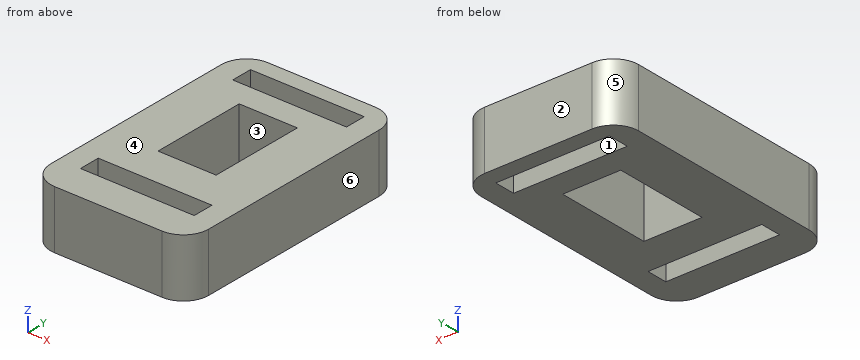
```python
from build123d import *

# Parameters (mm, degrees)
F1_DEPTH = 5.842
F2_W     = 5.842
F2_H     = 9.6774
F2_W_2   = 11.43
F2_H_2   = 2.116666
F2_H_3   = 2.116667
F3_DEPTH = 5.842


with BuildPart() as f1:
    # F0 (on Top) → F1 (new body)
    with BuildSketch(Plane.XY):
        with BuildLine():
            Line((4.632767, -11.371723), (-6.162233, -11.371723))
            ThreePointArc((-6.162233, -11.371723), (-7.958284, -12.115671), (-8.702233, -13.911723))
            Line((-8.702233, -13.911723), (-8.702233, -34.231723))
            ThreePointArc((-8.702233, -34.231723), (-7.958284, -36.027774), (-6.162233, -36.771723))
            Line((-6.162233, -36.771723), (4.632767, -36.771723))
            ThreePointArc((4.632767, -36.771723), (6.428818, -36.027774), (7.172767, -34.231723))
            Line((7.172767, -34.231723), (7.172767, -13.911723))
            ThreePointArc((7.172767, -13.911723), (6.428818, -12.115671), (4.632767, -11.371723))
        make_face()
    extrude(amount=-F1_DEPTH)

    # F2 (on Top) → F3 (cut, through all)
    with BuildSketch(Plane.XY):
        with Locations((-0.764733, -22.560423)):
            Rectangle(F2_W, F2_H)
        with Locations((-0.764733, -32.267456)):
            Rectangle(F2_W_2, F2_H_2)
        with Locations((-0.764733, -14.12339)):
            Rectangle(F2_W_2, F2_H_3)
    extrude(amount=-F3_DEPTH, mode=Mode.SUBTRACT)


solid = f1.part
```
The model under review builds one solid part; all positions refer to its coordinate system, in mm. Face numbers are marked on the shaded views. A direction names the side the tool comes from. Round coordinates to 2 decimals unless told otherwise and drop trailing zeros. Order: outer loops, then holes, each group sorted by start corner. A loop starts at its lowest first (then second) coordinate and runs counter-clockwise, first axis right, second up. Notation, with made-up numbers: (28.25, 89) - (78.25, 89) arc R18 cw to (78.25, 120) - close; hole circle Ø3 at (40, 45.5). An arc over 180 degrees is marked (long way). Answer in a Markdown table with one row per item.
(1) Machinability: for the marked faces 1 and 2, which of the approach directions +Z, -Z, +X, -X, +Y, -Y give a long, thin tool a straight path to every point of the face, cutting with its end or side? Answer none if there is none.
Result set:
| item | result |
|---|---|
| face 1 | +Z, -Z |
| face 2 | +Z, -Z, +X, -X, +Y |
(2) Take a section at A-A on y = -14.5. Write out the cut boundary in (x, z).
Result set:
| item | result |
|---|---|
| outline | (-8.7, -5.84) - (-6.48, -5.84) - (-6.48, 0) - (-8.7, 0) - close; (4.95, -5.84) - (7.17, -5.84) - (7.17, 0) - (4.95, 0) - close |
(3) Take a section at D-D on x = 3.5. Write out the cut boundary in (y, z), plus the area to 3 significant figures.
Result set:
| item | result |
|---|---|
| outline | (-36.77, -5.84) - (-33.33, -5.84) - (-33.33, 0) - (-36.77, 0) - close; (-31.21, -5.84) - (-15.18, -5.84) - (-15.18, 0) - (-31.21, 0) - close; (-13.07, -5.84) - (-11.37, -5.84) - (-11.37, 0) - (-13.07, 0) - close |
| area | 124 mm2 |
(4) Take a section at C-C on z = -0.35. Write out the cut boundary in (x, y), plus the area to 3 significant figures.
Result set:
| item | result |
|---|---|
| outline | (-8.7, -34.23) arc R2.54 ccw to (-6.16, -36.77) - (4.63, -36.77) arc R2.54 ccw to (7.17, -34.23) - (7.17, -13.91) arc R2.54 ccw to (4.63, -11.37) - (-6.16, -11.37) arc R2.54 ccw to (-8.7, -13.91) - close; hole (-6.48, -33.33) - (4.95, -33.33) - (4.95, -31.21) - (-6.48, -31.21) - close; hole (-6.48, -15.18) - (4.95, -15.18) - (4.95, -13.07) - (-6.48, -13.07) - close; hole (-3.69, -27.4) - (2.16, -27.4) - (2.16, -17.72) - (-3.69, -17.72) - close |
| area | 293 mm2 |
(5) Clearance check with a flat-ended pin moving along its axis: P1, Ø1.5, axis at x = -3.5, y = -20.5, coming from the +Z side. State where the tip first meets the part, or that it passes through.
Result set:
| item | result |
|---|---|
| P1 | stops at z = 0 |
(6) For line 1 (Y direction, x = 2.75, z = -0.3); line 2 (Y direction, x = -3.25, z = -0.4); line 3 (X direction, y = -20.5, z = -5.25), list the stretches that pass through material, from the lowest coordinate up. Write a range as from..to.
Result set:
| item | result |
|---|---|
| line 1 | y = -36.77..-33.33, -31.21..-15.18, -13.07..-11.37 |
| line 2 | y = -36.77..-33.33, -31.21..-27.4, -17.72..-15.18, -13.07..-11.37 |
| line 3 | x = -8.7..-3.69, 2.16..7.17 |
(7) Take a section at B-B on x = -1. Write out the cut boundary in (y, z).
Result set:
| item | result |
|---|---|
| outline | (-36.77, -5.84) - (-33.33, -5.84) - (-33.33, 0) - (-36.77, 0) - close; (-31.21, -5.84) - (-27.4, -5.84) - (-27.4, 0) - (-31.21, 0) - close; (-17.72, -5.84) - (-15.18, -5.84) - (-15.18, 0) - (-17.72, 0) - close; (-13.07, -5.84) - (-11.37, -5.84) - (-11.37, 0) - (-13.07, 0) - close |
(8) Mouldability with a two-part tool opening along X and no side actions: class the marked faces 3, 4, 5 and 6 as released by +X, released by -X, zero draft, split by the parting line, or undercut.
Result set:
| item | result |
|---|---|
| face 3 | undercut |
| face 4 | zero draft |
| face 5 | released by -X |
| face 6 | released by +X |
